Geometry check sheet. Reference: the model listing, model coordinates, mm. Coordinates: 2 decimals unless noted, no trailing zeros. Write each loop counter-clockwise with the first axis right and the second up, starting at its lowest first coordinate (ties: lowest second). Pieces come first, ordered by that corner, then holes.
from build123d import *

# Parameters (mm, degrees)
SKETCH1_R           = 4.25
BOSS_EXTRUDE1_DEPTH = 3.7
FILLET1_R           = 5


with BuildPart() as part:
    # Sketch1 → Boss-Extrude1 (new body)
    with BuildSketch(Plane(origin=(0, 0, 0), x_dir=(1, 0, 0), z_dir=(0, 1, 0))):
        with BuildLine():
            Line((37.5, -116), (37.5, 89))
            Line((37.5, 89), (-73, 89))
            ThreePointArc((-73, 89), (-76.535533906, 87.535533906), (-78, 84))
            Line((-78, 84), (-78, -111))
            ThreePointArc((-78, -111), (-76.535533906, -114.535533906), (-73, -116))
            Line((-73, -116), (37.5, -116))
        make_face()
        with Locations(Location((-50, -100, 0), (0, 0, 270))):
            Circle(SKETCH1_R, mode=Mode.SUBTRACT)
        with Locations(Location((-50, -75, 0), (0, 0, 270))):
            Circle(SKETCH1_R, mode=Mode.SUBTRACT)
        with Locations(Location((-25, -100, 0), (0, 0, 270))):
            Circle(SKETCH1_R, mode=Mode.SUBTRACT)
        with Locations(Location((-25, -75, 0), (0, 0, 270))):
            Circle(SKETCH1_R, mode=Mode.SUBTRACT)
        with Locations(Location((0, -100, 0), (0, 0, 270))):
            Circle(SKETCH1_R, mode=Mode.SUBTRACT)
        with Locations(Location((0, -75, 0), (0, 0, 270))):
            Circle(SKETCH1_R, mode=Mode.SUBTRACT)
        with Locations(Location((-50, -50, 0), (0, 0, 270))):
            Circle(SKETCH1_R, mode=Mode.SUBTRACT)
        with Locations(Location((-50, -25, 0), (0, 0, 270))):
            Circle(SKETCH1_R, mode=Mode.SUBTRACT)
        with Locations(Location((-25, -50, 0), (0, 0, 270))):
            Circle(SKETCH1_R, mode=Mode.SUBTRACT)
        with Locations(Location((0, -50, 0), (0, 0, 270))):
            Circle(SKETCH1_R, mode=Mode.SUBTRACT)
        with Locations(Location((-25, -25, 0), (0, 0, 270))):
            Circle(SKETCH1_R, mode=Mode.SUBTRACT)
        with Locations(Location((0, -25, 0), (0, 0, 270))):
            Circle(SKETCH1_R, mode=Mode.SUBTRACT)
        with Locations(Location((25, -100, 0), (0, 0, 270))):
            Circle(SKETCH1_R, mode=Mode.SUBTRACT)
        with Locations(Location((25, -75, 0), (0, 0, 270))):
            Circle(SKETCH1_R, mode=Mode.SUBTRACT)
        with Locations(Location((25, -50, 0), (0, 0, 270))):
            Circle(SKETCH1_R, mode=Mode.SUBTRACT)
        with Locations(Location((25, -25, 0), (0, 0, 270))):
            Circle(SKETCH1_R, mode=Mode.SUBTRACT)
        with Locations(Location((-50, 0, 0), (0, 0, 270))):
            Circle(SKETCH1_R, mode=Mode.SUBTRACT)
        with Locations(Location((-50, 25, 0), (0, 0, 270))):
            Circle(SKETCH1_R, mode=Mode.SUBTRACT)
        with Locations(Location((-25, 0, 0), (0, 0, 270))):
            Circle(SKETCH1_R, mode=Mode.SUBTRACT)
        with Locations(Location((0, 0, 0), (0, 0, 270))):
            Circle(SKETCH1_R, mode=Mode.SUBTRACT)
        with Locations(Location((-25, 25, 0), (0, 0, 270))):
            Circle(SKETCH1_R, mode=Mode.SUBTRACT)
        with Locations(Location((0, 25, 0), (0, 0, 270))):
            Circle(SKETCH1_R, mode=Mode.SUBTRACT)
        with Locations(Location((-50, 50, 0), (0, 0, 270))):
            Circle(SKETCH1_R, mode=Mode.SUBTRACT)
        with Locations(Location((-50, 75, 0), (0, 0, 270))):
            Circle(SKETCH1_R, mode=Mode.SUBTRACT)
        with Locations(Location((-25, 50, 0), (0, 0, 270))):
            Circle(SKETCH1_R, mode=Mode.SUBTRACT)
        with Locations(Location((-25, 75, 0), (0, 0, 270))):
            Circle(SKETCH1_R, mode=Mode.SUBTRACT)
        with Locations(Location((0, 50, 0), (0, 0, 270))):
            Circle(SKETCH1_R, mode=Mode.SUBTRACT)
        with Locations(Location((0, 75, 0), (0, 0, 270))):
            Circle(SKETCH1_R, mode=Mode.SUBTRACT)
        with Locations(Location((25, 0, 0), (0, 0, 270))):
            Circle(SKETCH1_R, mode=Mode.SUBTRACT)
        with Locations(Location((25, 25, 0), (0, 0, 270))):
            Circle(SKETCH1_R, mode=Mode.SUBTRACT)
        with Locations(Location((25, 50, 0), (0, 0, 270))):
            Circle(SKETCH1_R, mode=Mode.SUBTRACT)
        with Locations(Location((25, 75, 0), (0, 0, 270))):
            Circle(SKETCH1_R, mode=Mode.SUBTRACT)
    extrude(amount=BOSS_EXTRUDE1_DEPTH)

    # Fillet1
    fillet1_edges = [part.edges().sort_by_distance(p)[0] for p in [
        (37.5, 1.85, -89),
        (37.5, 1.85, 116),
    ]]
    fillet(fillet1_edges, radius=FILLET1_R)


solid = part.part
1. Sectioned sample at B-B, the plane x = 0. Give the number of separate pieces and of enclosed holes in the cut face, and give its area (3 significant figures).
Computed values:
separate pieces: 9
enclosed holes: 0
area: 507 mm2
2. Draft check along X on faces 1 (the cylindrical face through (-77, 2, 114)), 2 (the flat face through (-21, 3.7, 12)), 3 (the cylindrical face through (-51.628, 1.824, 78.926)). Enter one of: released by +X, released by -X, zero draft, split by the parting line, or undercut.
Computed values:
face 1: released by -X
face 2: zero draft
face 3: undercut
3. Sectioned sample at A-A, the plane z = -50. Record the boundary of the cut face in (x, y), and give its area (3 significant figures).
Computed values:
outline: (-78, 0) - (-54.25, 0) - (-54.25, 3.7) - (-78, 3.7) - close; (-45.75, 0) - (-29.25, 0) - (-29.25, 3.7) - (-45.75, 3.7) - close; (-20.75, 0) - (-4.25, 0) - (-4.25, 3.7) - (-20.75, 3.7) - close; (4.25, 0) - (20.75, 0) - (20.75, 3.7) - (4.25, 3.7) - close; (29.25, 0) - (37.5, 0) - (37.5, 3.7) - (29.25, 3.7) - close
area: 302 mm2
4. Thickness scan on line 1 along X through (y, z) = (1.1, -50); line 2 along X through (y, z) = (3.3, 72). Record the ranges inside material, lowest first.
Computed values:
line 1: x = -78 to -54.25, -45.75 to -29.25, -20.75 to -4.25, 4.25 to 20.75, 29.25 to 37.5
line 2: x = -78 to -53.01, -46.99 to -28.01, -21.99 to -3.01, 3.01 to 21.99, 28.01 to 37.5
